Check sheet for the drawn part. Datum: minimum x, y, z corner. Units: mm. A direction names the side the tool comes from. Give positions to 0.01 mm unless a question says otherwise; leave off trailing zeros. Loops run counter-clockwise (first coordinate to the right, second up) from the corner with the lowest first, then second, coordinate; pieces in that order, holes last.
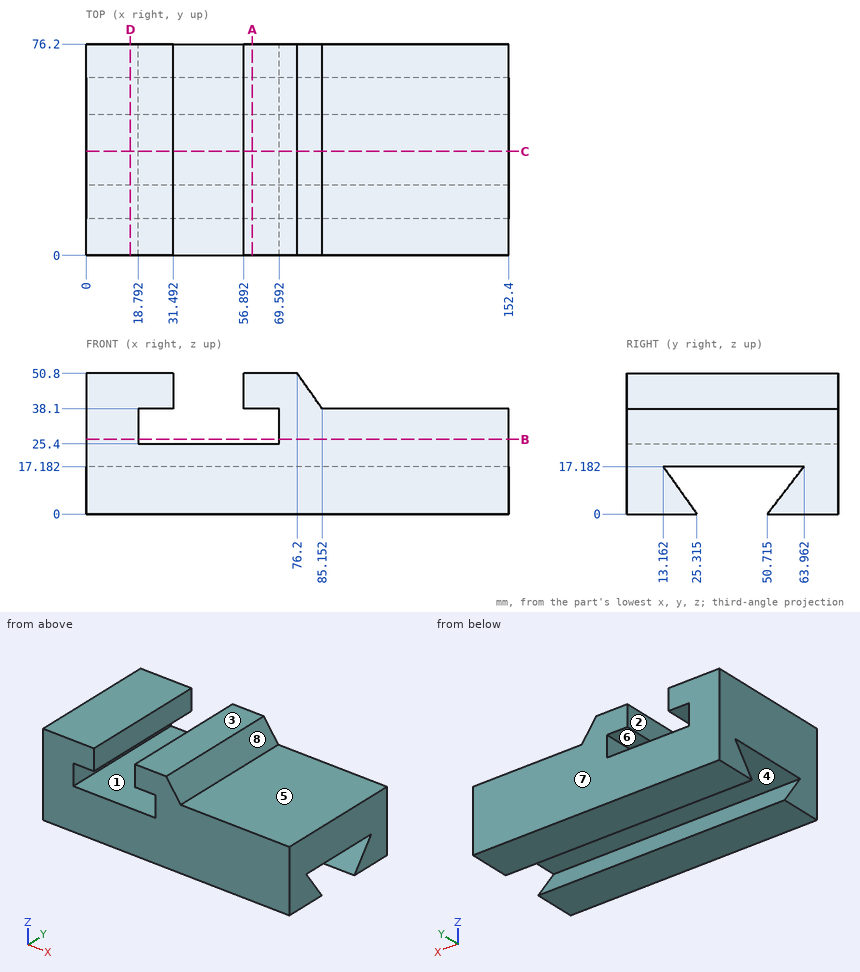
(1) Section check C-C on y = 37.5. Record the boundary of the cut face in (x, z).
(2) Release check for a two-part mould opening along X. For the marked faces 6, 7 and 8 record: pulls with the +X half, pulls with the -X half, needs draft (parallel to the pull), parting line crosses it, or undercut.
(3) Access from +Z, -Z, +X, -X, +Y, -Y to the whole of each face (thin tool, end or side, straight path). Record for the marked faces 1, 2, 3, 4 and 5.
(4) Material ranges on line 1 (Z direction, x = 30, y = 69.5); line 2 (Z direction, x = 60, y = 41.5); line 3 (Z direction, x = 49.5, y = 26), recorded low to high.
(5) Section check A-A on x = 60. Record the boundary of the cut face in (y, z) (1 decimal), plus the area to 3 significant figures.
(6) Section check B-B on z = 27. Record the boundary of the cut face in (x, y).
(7) Section check D-D on x = 16. Record the boundary of the cut face in (y, z) (1 decimal).
(8) Gauge pin test, flat ends, axial feed: pin 1 Ø3 at (x, z) = (77.5, 22.5) entering from -Y; pin 2 Ø10 at (y, z) = (24, 46) entering from +X; pin 3 Ø6 at (x, y) = (100.5, 29) entering from -Z. Record the tip position at first contact, or that the pin passes through.
Computed values:
1. outline: (0, 17.18) - (152.4, 17.18) - (152.4, 38.1) - (85.15, 38.1) - (76.2, 50.8) - (56.89, 50.8) - (56.89, 38.1) - (69.59, 38.1) - (69.59, 25.4) - (18.79, 25.4) - (18.79, 38.1) - (31.49, 38.1) - (31.49, 50.8) - (0, 50.8) - close
2. face 6: undercut
2. face 7: needs draft
2. face 8: pulls with the +X half
3. face 1: +Y, -Y
3. face 2: +Z, +Y, -Y
3. face 3: +Z, +X, -X, +Y, -Y
3. face 4: +X, -X
3. face 5: +Z, +X, +Y, -Y
4. line 1: z = 0 to 25.4, 38.1 to 50.8
4. line 2: z = 17.18 to 25.4, 38.1 to 50.8
4. line 3: z = 17.18 to 25.4
5. outline: (0, 0) - (25.3, 0) - (13.2, 17.2) - (64, 17.2) - (50.7, 0) - (76.2, 0) - (76.2, 25.4) - (0, 25.4) - close; (0, 38.1) - (76.2, 38.1) - (76.2, 50.8) - (0, 50.8) - close
5. area: 2,250 mm2
6. outline: (0, 0) - (18.79, 0) - (18.79, 76.2) - (0, 76.2) - close; (69.59, 0) - (152.4, 0) - (152.4, 76.2) - (69.59, 76.2) - close
7. outline: (0, 0) - (25.3, 0) - (13.2, 17.2) - (64, 17.2) - (50.7, 0) - (76.2, 0) - (76.2, 50.8) - (0, 50.8) - close
8. pin 1: stops at y = 0
8. pin 2: stops at x = 83.11
8. pin 3: stops at z = 17.18
